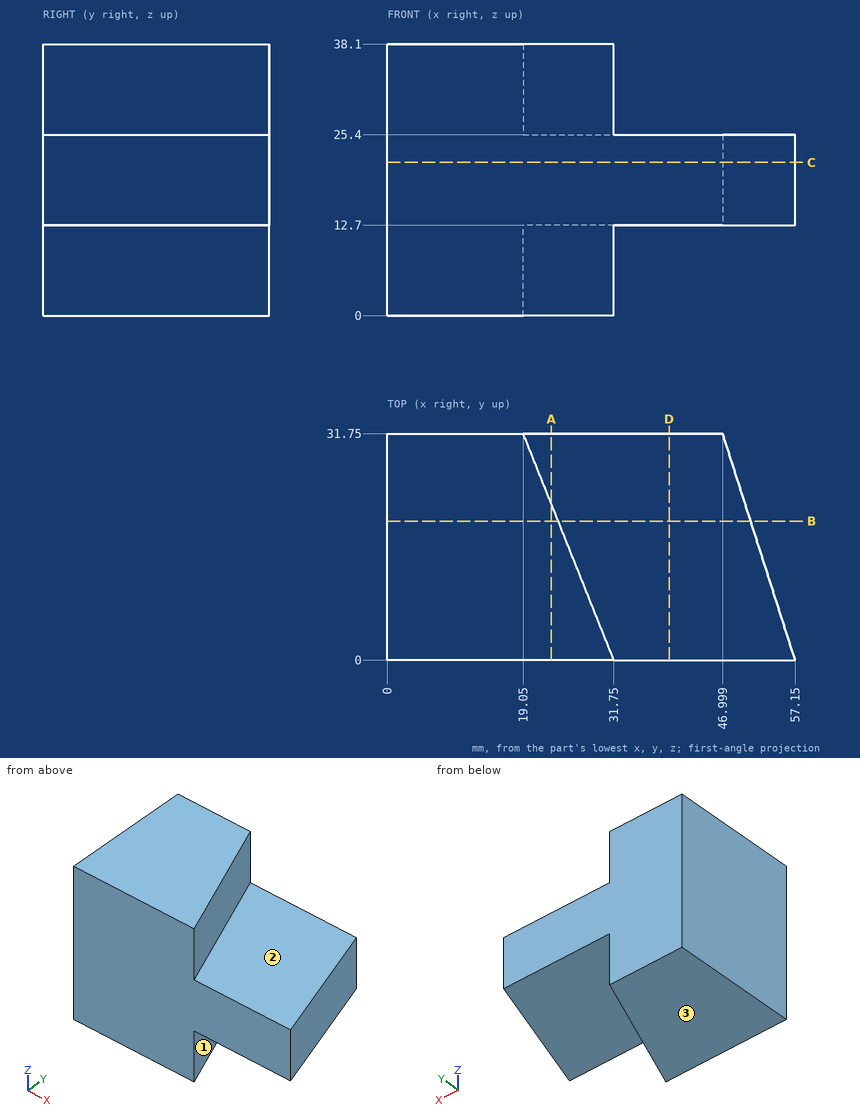
Here's the drawing with two shaded views (mm, measured from the low corner). I have some questions. A direction names the side the tool comes from. Coordinates: 2 decimals unless noted, no trailing zeros. Write each loop counter-clockwise with the first axis right and the second up, starting at its lowest first coordinate (ties: lowest second). Pieces come first, ordered by that corner, then holes. Notation, with made-up numbers: (-1.5, 25.5) -> (4.5, 25.5) arc R30 cw to (4.5, 48.5) -> close; hole circle Ø3 at (0.5, 85). An arc over 180 degrees is marked (long way). Use a Markdown table: item, result. Add a question column.
(1) If we section it at C-C, the plane z = 21.5: Write out the boundary of the cut face in (x, y), and give its area (3 significant figures).
(2) I'm going to push flat-ended pins straight in: P1, Ø5, axis at y = 10.5, z = 13, coming from the +X side; P2, Ø9.5, axis at x = 45, y = 21, coming from the -Z side; P3, Ø3, axis at y = 3.5, z = 9, coming from the +X side. Where does each tip first touch, or does it pass through?
(3) If we section it at B-B, the plane y = 19.5: Write out the boundary of the cut face in (x, z), and give its area (4 significant figures).
(4) If we section it at D-D, the plane x = 39.5: Write out the boundary of the cut face in (y, z), and give its area (3 significant figures).
(5) For the marked faces 1, 2 and 3, which set-ups out of +Z, -Z, +X, -X, +Y, -Y let a thin tool reach every point of the face, with its end or its side?
(6) If we section it at A-A, the plane x = 23: Write out the boundary of the cut face in (y, z) (3 decimals).
(7) Please list where these lines run through material, in increasing order: line 1 (Z direction, x = 50, y = 21.5); line 2 (X direction, y = 4, z = 5); line 3 (X direction, y = 24, z = 9).
Outcome:
| question | item | result |
|---|---|---|
| 1 | outline | (0, 0) -> (57.15, 0) -> (47, 31.75) -> (0, 31.75) -> close |
| 1 | area | 1,650 mm^2 |
| 2 | P1 | stops at x = 54.59 |
| 2 | P2 | stops at z = 12.7 |
| 2 | P3 | stops at x = 30.95 |
| 3 | outline | (0, 0) -> (23.95, 0) -> (23.95, 12.7) -> (50.92, 12.7) -> (50.92, 25.4) -> (23.95, 25.4) -> (23.95, 38.1) -> (0, 38.1) -> close |
| 3 | area | 1,255 mm^2 |
| 4 | outline | (0, 12.7) -> (31.75, 12.7) -> (31.75, 25.4) -> (0, 25.4) -> close |
| 4 | area | 403 mm^2 |
| 5 | face 1 | -Z, +X, +Y |
| 5 | face 2 | +Z, +X, +Y |
| 5 | face 3 | -Z, +X, -X, +Y, -Y |
| 6 | outline | (0, 0) -> (21.875, 0) -> (21.875, 12.7) -> (31.75, 12.7) -> (31.75, 25.4) -> (21.875, 25.4) -> (21.875, 38.1) -> (0, 38.1) -> close |
| 7 | line 1 | z = 12.7 to 25.4 |
| 7 | line 2 | x = 0 to 30.15 |
| 7 | line 3 | x = 0 to 22.15 |
